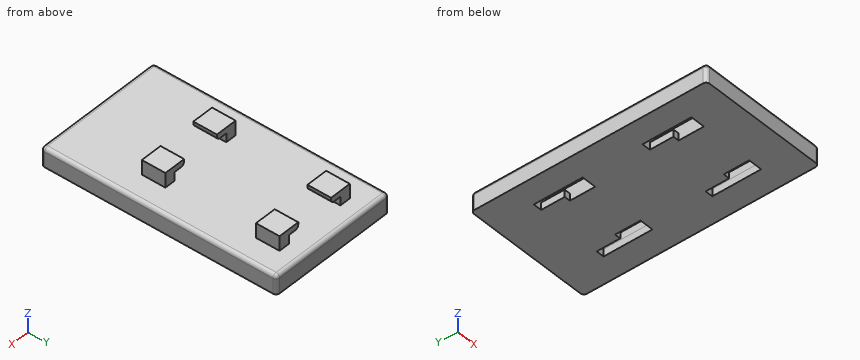
from build123d import *

# Parameters (mm, degrees)
SKETCH_W        = 36
SKETCH_H        = 65
PAD_DEPTH       = 2.2
POCKET_DEPTH    = 2.201
SKETCH002_W     = 36
SKETCH002_H     = 65
PAD001_DEPTH    = 3
POCKET001_START = 2
SKETCH003_W     = 4
SKETCH003_H     = 13.5
SKETCH003_W_2   = 3.848829
POCKET001_DEPTH = 2
SKETCH004_W     = 6
SKETCH004_H     = 6.5
PAD002_DEPTH    = 4
SKETCH005_W     = 16.5
SKETCH005_H     = 38
POCKET002_DEPTH = 2.4
FILLET_R        = 1
FILLET001_R     = 1
FILLET002_R     = 1
FILLET003_R     = 1
FILLET004_R     = 1
FILLET005_R     = 1


with BuildPart() as part:
    # Sketch → Pad (new body)
    with BuildSketch(Plane.XY):
        Rectangle(SKETCH_W, SKETCH_H)
    extrude(amount=PAD_DEPTH)

    # Sketch001 → Pocket (cut, through all)
    with BuildSketch(Plane.XY):
        Polygon((-11.25, -9), (-11.25, -22.5), (-7.25, -22.5), (-7.25, -15.5), (-8.9, -15.5), (-8.9, -9), align=None)
        Polygon((-11.25, 21), (-11.25, 7.5), (-7.25, 7.5), (-7.25, 14.5), (-8.9, 14.5), (-8.9, 21), align=None)
        Polygon((11.098829, -9), (11.098829, -22.5), (7.25, -22.5), (7.25, -15.5), (8.977746, -15.5), (8.977746, -9), align=None)
        Polygon((11.098829, 21), (11.098829, 7.5), (7.25, 7.5), (7.25, 14.5), (8.903816, 14.5), (8.903816, 21), align=None)
    extrude(amount=POCKET_DEPTH, mode=Mode.SUBTRACT)

    # Sketch002 (on Face5 of Pocket) → Pad001 (join)
    with BuildSketch(Plane.XY.offset(2.2)):
        Rectangle(SKETCH002_W, SKETCH002_H)
    extrude(amount=PAD001_DEPTH)

    # Sketch003 → Pocket001 (cut)
    with BuildSketch(Plane.XY.offset(POCKET001_START)):
        with Locations((-9.25, 14.25)):
            Rectangle(SKETCH003_W, SKETCH003_H)
        with Locations((9.174415, 14.25)):
            Rectangle(SKETCH003_W_2, SKETCH003_H)
        with Locations((9.174415, -15.75)):
            Rectangle(SKETCH003_W_2, SKETCH003_H)
        with Locations((-9.25, -15.75)):
            Rectangle(SKETCH003_W, SKETCH003_H)
    extrude(amount=POCKET001_DEPTH, mode=Mode.SUBTRACT)

    # Sketch004 (on Face33 of Pocket001) → Pad002 (join)
    with BuildSketch(Plane.XY.offset(5.2)):
        with Locations((-8.25, 24.25)):
            Rectangle(SKETCH004_W, SKETCH004_H)
        with Locations((8.25, 24.25)):
            Rectangle(SKETCH004_W, SKETCH004_H)
        with Locations((-8.25, -7.25)):
            Rectangle(SKETCH004_W, SKETCH004_H)
        with Locations((8.25, -7.25)):
            Rectangle(SKETCH004_W, SKETCH004_H)
    extrude(amount=PAD002_DEPTH)

    # Sketch005 (on Face33 of Pad002) → Pocket002 (cut)
    with BuildSketch(Plane.XY.offset(5.2)):
        with Locations((0, 8.5)):
            Rectangle(SKETCH005_W, SKETCH005_H)
    extrude(amount=POCKET002_DEPTH, mode=Mode.SUBTRACT)

    # Fillet
    fillet_edges = [part.edges().sort_by_distance(p)[0] for p in [
        (18, 0, 5.2),
    ]]
    fillet(fillet_edges, radius=FILLET_R)

    # Fillet001
    fillet001_edges = [part.edges().sort_by_distance(p)[0] for p in [
        (-0.5, -32.5, 5.2),
    ]]
    fillet(fillet001_edges, radius=FILLET001_R)

    # Fillet002
    fillet002_edges = [part.edges().sort_by_distance(p)[0] for p in [
        (-18, 0.5, 5.2),
    ]]
    fillet(fillet002_edges, radius=FILLET002_R)

    # Fillet003
    fillet003_edges = [part.edges().sort_by_distance(p)[0] for p in [
        (0, 32.5, 5.2),
    ]]
    fillet(fillet003_edges, radius=FILLET003_R)

    # Fillet004
    fillet004_edges = [part.edges().sort_by_distance(p)[0] for p in [
        (5.25, -7.25, 7.6),
        (5.25, 24.25, 7.6),
    ]]
    fillet(fillet004_edges, radius=FILLET004_R)

    # Fillet005
    fillet005_edges = [part.edges().sort_by_distance(p)[0] for p in [
        (-5.25, 24.25, 7.6),
        (-5.25, -7.25, 7.6),
    ]]
    fillet(fillet005_edges, radius=FILLET005_R)


solid = part.part
Could you check a few things on this model? Use its own coordinates, in mm. Coordinates: 2 decimals unless noted, no trailing zeros. Order: outer loops, then holes, each group sorted by start corner. A loop starts at its lowest first (then second) coordinate and runs counter-clockwise, first axis right, second up. Notation, with made-up numbers: (-38, 11.25) -> (-12, 11.25) arc R9 ccw to (-12, 21.25) -> close; hole circle Ø5 at (7.5, 7.5). An arc over 180 degrees is marked (long way). One line per item, written item: value. Start each with the question number.
1) I'm going to push flat-ended pins straight in: pin 1 (8 mm diameter, centred on x = 0, y = -22, fed in from +Z); pin 2 (1.2 mm diameter, centred on x = -7.5, z = 6.5, fed in from -Y); pin 3 (3 mm diameter, centred on x = -9, z = 7.5, fed in from +Y); pin 4 (0.5 mm diameter, centred on y = 23, z = 9, fed in from +X). Where does each tip first touch, or does it pass through?
2) Imagine slicing it at D-D on y = 2.5. List the corners of the cut face in (x, z) for me, plus the area to 3 significant figures.
3) Imagine slicing it at A-A on z = 6.5. List the corners of the cut face in (x, y) for me.
4) Imagine slicing it at B-B on y = 25. List the corners of the cut face in (x, z) for me.
5) Imagine slicing it at C-C on x = -9.5. List the corners of the cut face in (y, z) for me, plus the area to 3 significant figures.
6) If I drill on L1, parallel to X at y = -20, z = 2.5; L2, parallel to Y at x = 11, z = 3; L3, parallel to Y at x = 11, z = 5.5, over which ranges is the centre line in solid material (lowest first)? Write a range as [from, to].
Answer list:
1. pin 1: stops at z = 5.2
1. pin 2: passes through
1. pin 3: stops at y = 27.5
1. pin 4: stops at x = 11.25
2. outline: (-18, 0) -> (18, 0) -> (18, 4.2) arc R1 ccw to (17, 5.2) -> (-17, 5.2) arc R1 ccw to (-18, 4.2) -> close
2. area: 187 mm2
3. outline: (-11.25, -10.5) -> (-8.25, -10.5) -> (-8.25, -4) -> (-11.25, -4) -> close; (-11.25, 21) -> (-8.25, 21) -> (-8.25, 27.5) -> (-11.25, 27.5) -> close; (8.25, -10.5) -> (11.25, -10.5) -> (11.25, -4) -> (8.25, -4) -> close; (8.25, 21) -> (11.25, 21) -> (11.25, 27.5) -> (8.25, 27.5) -> close
4. outline: (-18, 0) -> (18, 0) -> (18, 4.2) arc R1 ccw to (17, 5.2) -> (11.25, 5.2) -> (11.25, 9.2) -> (5.25, 9.2) -> (5.25, 8.6) arc R1 ccw to (6.25, 7.6) -> (8.25, 7.6) -> (8.25, 5.2) -> (-8.25, 5.2) -> (-8.25, 7.6) -> (-6.25, 7.6) arc R1 ccw to (-5.25, 8.6) -> (-5.25, 9.2) -> (-11.25, 9.2) -> (-11.25, 5.2) -> (-17, 5.2) arc R1 ccw to (-18, 4.2) -> close
5. outline: (-32.5, 0) -> (-22.5, 0) -> (-22.5, 4) -> (-9, 4) -> (-9, 0) -> (7.5, 0) -> (7.5, 4) -> (21, 4) -> (21, 0) -> (32.5, 0) -> (32.5, 4.2) arc R1 ccw to (31.5, 5.2) -> (27.5, 5.2) -> (27.5, 9.2) -> (21, 9.2) -> (21, 5.2) -> (-4, 5.2) -> (-4, 9.2) -> (-10.5, 9.2) -> (-10.5, 5.2) -> (-31.5, 5.2) arc R1 ccw to (-32.5, 4.2) -> close
5. area: 282 mm2
6. L1: x = [-18, -11.25], [-7.25, 7.25], [11.1, 18]
6. L2: y = [-32.5, -22.5], [-9, 7.5], [21, 32.5]
6. L3: y = [-10.5, -4], [21, 27.5]
